Input: part model. Units: mm. Frame: model coordinates. A direction names the side the tool comes from. Give positions to 0.01 mm unless a question says otherwise; leave off trailing zeros. Write each loop counter-clockwise with the first axis right and the second up, starting at its lowest first coordinate (ties: lowest second). Pieces come first, ordered by that corner, then holes.
```python
from build123d import *

# Parameters (mm, degrees)
F0_R     = 3
F1_DEPTH = 5


with BuildPart() as f1:
    # F0 (on Top) → F1 (new body)
    with BuildSketch(Plane.XY):
        Polygon((30, -22.5), (30, 22.5), (11, 22.5), (6, 22.5), (-6, 22.5), (-11, 22.5), (-30, 22.5), (-30, -22.5), align=None)
        Polygon((-11, 22.5), (-6, 22.5), (-6, 27.5), align=None)
        with BuildLine():
            Line((-6, 22.5), (6, 22.5))
            Line((6, 22.5), (6, 27.5))
            Line((6, 27.5), (6, 32.5))
            ThreePointArc((6, 32.5), (0, 38.5), (-6, 32.5))
            Line((-6, 32.5), (-6, 27.5))
            Line((-6, 27.5), (-6, 22.5))
        make_face()
        with Locations((0, 32.5)):
            Circle(F0_R, mode=Mode.SUBTRACT)
        Polygon((6, 22.5), (11, 22.5), (6, 27.5), align=None)
    extrude(amount=F1_DEPTH)


solid = f1.part
```
Item 1: Section C-C (x = -20.5). Return loops of the section in (y, z).
Item 2: Set-up query: faces 1 (the flat face through (30, 0, 2)), 2 (the flat face through (-20, 22.5, 2)), 3 (the flat face through (21, 22.5, 2)). Return all of +Z, -Z, +X, -X, +Y, -Y with unobstructed straight access to the full face (end or side cutting, diameter ignored); none if empty.
Item 3: Mould query, pull axis X, two halves, no side actions, for faces 4 (the flat face through (0, 2, 5)), 5 (the cylindrical face through (0.1, 38.5, 2.5)), 6 (the flat face through (6, 30, 2)), 7 (the cylindrical face through (-2.21, 34.53, 2.46)). Classes: +X half, -X half, draft (parallel to the pull), parting line (faces both ways), or undercut.
Item 4: Pin query (flat end, axial travel): pin 1 (1.5 mm diameter, centred on y = 30, z = 3, fed in from -X); pin 2 (2.5 mm diameter, centred on y = 29.5, z = 3.5, fed in from +X); pin 3 (5.5 mm diameter, centred on x = 0, y = 32.5, fed in from +Z). Return the tip coordinate at first contact, or that it passes through.
Item 5: Section B-B (x = 0). Return loops of the section in (y, z).
Item 6: Section A-A (z = 3.7). Return loops of the section in (x, y), and give its area (3 significant figures).
Item 7: Ray query, line 1 (Y direction, x = 0, z = 2.4); line 2 (Y direction, x = 12, z = 1.35); line 3 (Y direction, x = -2.5, z = 2.7). Return the intervals inside material, ascending.
Solved:
1. outline: (-22.5, 0) - (22.5, 0) - (22.5, 5) - (-22.5, 5) - close
2. face 1: +Z, -Z, +X, +Y, -Y
2. face 2: +Z, -Z, -X, +Y
2. face 3: +Z, -Z, +X, +Y
3. face 4: draft
3. face 5: parting line
3. face 6: +X half
3. face 7: undercut
4. pin 1: stops at x = -6
4. pin 2: stops at x = 6
4. pin 3: passes through
5. outline: (-22.5, 0) - (29.5, 0) - (29.5, 5) - (-22.5, 5) - close; (35.5, 0) - (38.5, 0) - (38.5, 5) - (35.5, 5) - close
6. outline: (-30, -22.5) - (30, -22.5) - (30, 22.5) - (11, 22.5) - (6, 27.5) - (6, 32.5) arc R6 ccw to (-6, 32.5) - (-6, 27.5) - (-11, 22.5) - (-30, 22.5) - close; hole circle Ø6 at (0, 32.5)
6. area: 2,870 mm2
7. line 1: y = -22.5 to 29.5, 35.5 to 38.5
7. line 2: y = -22.5 to 22.5
7. line 3: y = -22.5 to 30.84, 34.16 to 37.95
